from build123d import *

# Parameters (mm, degrees)
SKETCH1_W           = 67.31
SKETCH1_H           = 41.91
BOSS_EXTRUDE5_DEPTH = 3.175
SKETCH2_W           = 67.31
SKETCH2_H           = 41.91
SKETCH2_W_2         = 60.96
SKETCH2_H_2         = 35.56
BOSS_EXTRUDE6_DEPTH = 7.62
SKETCH4_W           = 12.7
SKETCH4_H           = 6.35
SKETCH4_W_2         = 6.35
SKETCH4_H_2         = 12.7
BOSS_EXTRUDE8_DEPTH = 3.175
SKETCH6_R           = 1.5875
CUT_EXTRUDE1_DEPTH  = 50.62353348


with BuildPart() as part:
    # Sketch1 → Boss-Extrude5 (new body)
    with BuildSketch(Plane(origin=(0, 0, 0), x_dir=(1, 0, 0), z_dir=(0, 1, 0))):
        Rectangle(SKETCH1_W, SKETCH1_H)
    extrude(amount=BOSS_EXTRUDE5_DEPTH)

    # Sketch2 → Boss-Extrude6 (add)
    with BuildSketch(Plane(origin=(0, 3.175, 0), x_dir=(1, 0, 0), z_dir=(0, 1, 0))):
        Rectangle(SKETCH2_W, SKETCH2_H)
        Rectangle(SKETCH2_W_2, SKETCH2_H_2, mode=Mode.SUBTRACT)
    extrude(amount=BOSS_EXTRUDE6_DEPTH)

    # Sketch4 → Boss-Extrude8 (add)
    with BuildSketch(Plane(origin=(0, 10.795, 0), x_dir=(1, 0, 0), z_dir=(0, 1, 0))):
        with Locations((0, -24.13)):
            Rectangle(SKETCH4_W, SKETCH4_H)
        with Locations((0, 24.13)):
            Rectangle(SKETCH4_W, SKETCH4_H)
        with Locations((36.83, 0)):
            Rectangle(SKETCH4_W_2, SKETCH4_H_2)
        with Locations((-36.83, 0)):
            Rectangle(SKETCH4_W_2, SKETCH4_H_2)
    extrude(amount=-BOSS_EXTRUDE8_DEPTH)

    # Sketch6 → Cut-Extrude1 (cut, through all)
    with BuildSketch(Plane(origin=(0, 10.795, 0), x_dir=(1, 0, 0), z_dir=(0, 1, 0))):
        with BuildLine():
            ThreePointArc((0, 25.7175), (-1.5875, 24.13), (0, 22.5425))
            Line((0, 22.5425), (0, 25.7175))
        make_face()
        with BuildLine():
            Line((0, 25.7175), (0, 22.5425))
            ThreePointArc((0, 22.5425), (1.122532015, 23.007467985), (1.5875, 24.13))
            ThreePointArc((1.5875, 24.13), (1.122532015, 25.252532015), (0, 25.7175))
        make_face()
        with Locations(Location((-36.806414665, 0, 0), (0, 0, 270))):
            Circle(SKETCH6_R)
        with Locations(Location((36.83, 0, 0), (0, 0, 270))):
            Circle(SKETCH6_R)
        with Locations(Location((0, -24.13, 0), (0, 0, 270))):
            Circle(SKETCH6_R)
    extrude(amount=-CUT_EXTRUDE1_DEPTH, mode=Mode.SUBTRACT)


solid = part.part
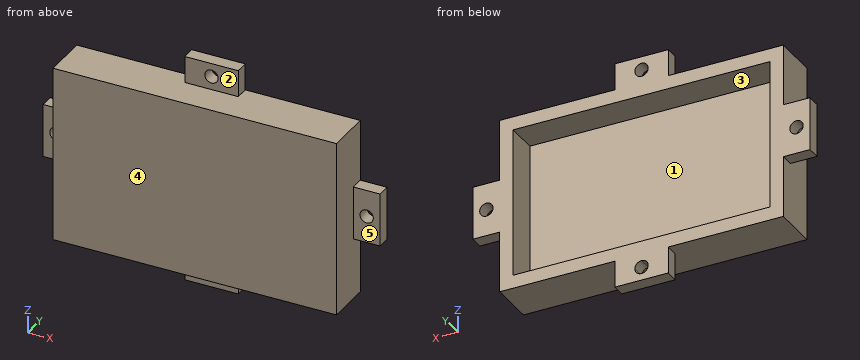
Source: CAD feature listing. Evaluate the final solid. Frame: model axes, mm. Face numbers are marked on the shaded views. A direction names the side the tool comes from. Coordinates: 2 decimals unless noted, no trailing zeros. Loops run counter-clockwise (first coordinate to the right, second up) from the corner with the lowest first, then second, coordinate; pieces in that order, holes last. Notation, with made-up numbers: (7.5, 36.5) - (35.5, 36.5) arc R19 cw to (35.5, 61.5) - close; hole circle Ø9 at (-33, -27). An arc over 180 degrees is marked (long way). Return JSON: item names as keys, results as strings.
Q1. Contact query for flat-ended pins moving along their axis: P1, Ø2.5, axis at x = -5.5, y = 5.5, coming from the -Z side (3 decimals); P2, Ø2, axis at x = -19.5, z = -6, coming from the +Y side (3 decimals); P3, Ø2.5, axis at x = 38, y = 8.5, coming from the +Z side; P4, Ø3, axis at x = 0, z = 24.13, coming from the +Y side. Output: stop coordinate, or through.
Results:
{"P1": "z = -20.955", "P2": "y = 3.175", "P3": "z = 6.35", "P4": "through"}
Q2. Material intervals for line 1 along X through (y, z) = (8.95, 0) (1 decimal); line 2 along X through (y, z) = (8, -3.5) (3 decimals); line 3 along X through (y, z) = (3.25, -14) (3 decimals), sorted ascending.
Results:
{"line 1": "-40 to -38.4, -35.2 to -30.5, 30.5 to 35.2, 38.4 to 40", "line 2": "-40.005 to -30.48, 30.48 to 40.005", "line 3": "-33.655 to -30.48, 30.48 to 33.655"}
Q3. Mould query, pull axis Z, two halves, no side actions, for the marked faces 1 and 2. Classes: released by +Z, released by -Z, zero draft, split by the parting line, or undercut.
Results:
{"face 1": "undercut", "face 2": "zero draft"}
Q4. Section B-B, the plane y = 5. Return loops of the section in (x, z) (3 decimals), plus the area to 3 significant figures.
Results:
{"outline": "(-33.655, -20.955) - (33.655, -20.955) - (33.655, 20.955) - (-33.655, 20.955) - close; hole (-30.48, -17.78) - (30.48, -17.78) - (30.48, 17.78) - (-30.48, 17.78) - close", "area": "653 mm2"}
Q5. Section C-C, the plane z = 0. Return loops of the section in (x, y) (1 decimal), plus the area to 3 significant figures.
Results:
{"outline": "(-40, 7.6) - (-38.4, 7.6) - (-38.4, 10.8) - (-40, 10.8) - close; (-35.2, 7.6) - (-33.7, 7.6) - (-33.7, 0) - (33.7, 0) - (33.7, 7.6) - (35.2, 7.6) - (35.2, 10.8) - (30.5, 10.8) - (30.5, 3.2) - (-30.5, 3.2) - (-30.5, 10.8) - (-35.2, 10.8) - close; (38.4, 7.6) - (40, 7.6) - (40, 10.8) - (38.4, 10.8) - close", "area": "282 mm2"}
Q6. Access query for the marked faces 3, 4 and 5. Directions: +Z, -Z, +X, -X, +Y, -Y. A direction counts if a zero-diameter tool reaches every point of the face in a straight line with its end or side. Return the directions, or none.
Results:
{"face 3": "+Y", "face 4": "+Z, -Z, +X, -X, -Y", "face 5": "+Z, -Z, +X, -Y"}
